The model under review builds one solid part; all positions refer to its coordinate system, in mm. A direction names the side the tool comes from. Round coordinates to 2 decimals unless told otherwise and drop trailing zeros. Write each loop counter-clockwise with the first axis right and the second up, starting at its lowest first coordinate (ties: lowest second). Pieces come first, ordered by that corner, then holes. Notation, with made-up numbers: M 74,13 L 95,13 A21 cw 95,28 Z; hole C 37,73 d3. An arc over 180 degrees is marked long. One line per item, written item: value. Start each with the question number.
1) For P1, Ø2, axis at y = -4, z = 2, coming from the -X side; P2, Ø1.5, axis at x = -11, z = 2, coming from the -Y side; P3, Ø1.5, axis at x = -20, z = 5, coming from the -Y side, all flat-tipped, find the tip position at first contact; note any pin that passes through.
2) Take a section at B-B, the plane y = -20.5. Write out the cut boundary in (x, z), and give its area (3 significant figures).
3) Take a section at D-D, the plane y = 13. Write out the cut boundary in (x, z), and give its area (3 significant figures).
4) Take a section at C-C, the plane z = 4. Write out the cut boundary in (x, y).
5) Wall thickness on probe 1 along X at (y, z) = (-19, 1.5); probe 2 along X at (y, z) = (-24.5, 5); probe 3 along Y at (x, z) = (0, 4.5): over which ranges is each line inside the solid? List them lowest first.
6) Mouldability with a two-part tool opening along Y and no side actions: class faces 1 (the face through (-3, -13, 7)), 2 (the face through (41.56, -23.91, 3.45)), 3 (the face through (-1.313, 29.172, 3.451)), 4 (the face through (15.219, -11.103, 3.451)) as +Y half, -Y half, draft (parallel to the pull), parting line (faces both ways), or undercut.
7) Take a section at A-A, the plane x = 16.5. Write out the cut boundary in (y, z), and give its area (3 significant figures).
8) Tool access review of faces 5 (the face through (13.575, 7.697, 3.451)), 6 (the face through (0.18, -10.75, 3.45)): name each direction out of +Z, -Z, +X, -X, +Y, -Y from which nothing blocks a thin tool from reaching the whole face with its end or side.
from build123d import *

# Parameters (mm, degrees)
F0_R        = 5.7
F1_DEPTH    = 7
F2_T1_DEPTH = 7


# Not quite as in the source:
# - a fillet or chamfer that OpenCascade refuses, or shapes differently, is made with other operations: its cross-section is extruded or revolved along the edge and cut away or added


with BuildPart() as f1:
    # F0 (on Top) → F1 (new body)
    with BuildSketch(Plane.XY):
        with BuildLine():
            ThreePointArc((35.7857254885, -10.7114257283), (13.3672908486, 8.0601420356), (8.7727432709, 36.9365701488))
            ThreePointArc((8.7727432709, 36.9365701488), (-0.3049324387, 47.9411231542), (-8.6164959528, 36.3470602301))
            ThreePointArc((-8.6164959528, 36.3470602301), (-13.6639331853, 7.5463424369), (-36.374379713, -10.8708665409))
            ThreePointArc((-36.374379713, -10.8708665409), (-41.3657643181, -24.2346408155), (-27.1692295357, -25.6356345017))
            ThreePointArc((-27.1692295357, -25.6356345017), (0.2966423367, -15.6064844725), (27.6016364421, -26.0657036079))
            ThreePointArc((27.6016364421, -26.0657036079), (41.6706967568, -23.7064823387), (35.7857254885, -10.7114257283))
        make_face()
        with Locations((-33.7284768728, -19.4731452019)):
            Circle(F0_R, mode=Mode.SUBTRACT)
        with Locations((33.7284768728, -19.4731452019)):
            Circle(F0_R, mode=Mode.SUBTRACT)
        with BuildLine():
            ThreePointArc((4.7464996897, 9.6453740568), (9.1265374503, 5.6805645994), (10.75, 0))
            ThreePointArc((10.75, 0), (10.7467864276, -0.2628335582), (10.7371476318, -0.5255099751))
            ThreePointArc((10.7371476318, -0.5255099751), (18.1244877352, -7.9521533479), (27.0404212358, -13.4506945549))
            ThreePointArc((27.0404212358, -13.4506945549), (26.0732155549, -14.7406010495), (25.3516724639, -16.1823781342))
            ThreePointArc((25.3516724639, -16.1823781342), (16.0918632419, -11.4192065952), (5.9798891173, -8.9332763388))
            ThreePointArc((5.9798891173, -8.9332763388), (0.0934488338, -10.749593821), (-5.8236788043, -9.0358876257))
            ThreePointArc((-5.8236788043, -9.0358876257), (-15.9490106817, -11.7201901353), (-25.168853801, -16.6923444418))
            ThreePointArc((-25.168853801, -16.6923444418), (-25.8023427534, -15.2097665041), (-26.6901867898, -13.864003315))
            ThreePointArc((-26.6901867898, -13.864003315), (-17.9352546235, -8.2263590641), (-10.726388807, -0.712097718))
            ThreePointArc((-10.726388807, -0.712097718), (-9.3561457462, 5.2938678465), (-4.9134688275, 9.5613976008))
            ThreePointArc((-4.9134688275, 9.5613976008), (-2.1754770535, 19.6723434832), (-1.8715674348, 30.1430389967))
            ThreePointArc((-1.8715674348, 30.1430389967), (-0.2708728015, 29.9503675537), (1.3385143259, 30.0463814492))
            ThreePointArc((1.3385143259, 30.0463814492), (1.8433913815, 19.6455656593), (4.7464996897, 9.6453740568))
        make_face(mode=Mode.SUBTRACT)
        with Locations((0, 38.9462904038)):
            Circle(F0_R, mode=Mode.SUBTRACT)
    extrude(amount=F1_DEPTH)

    # F2: fillet of radius 2 on 6 edges, made by hand

    # F2_s2 → F2_t1 (join)
    with BuildSketch(Plane.XY):
        with BuildLine():
            ThreePointArc((1.2437301381, 27.9302712072), (0.7204204263, 29.321617428), (-0.6184050998, 29.9675613661))
            ThreePointArc((-0.6184050998, 29.9675613661), (0.362205019, 29.9535818283), (1.3385143259, 30.0463814492))
            ThreePointArc((1.3385143259, 30.0463814492), (1.278556326, 28.9888891766), (1.2437301381, 27.9302712072))
        make_face()
        with BuildLine():
            ThreePointArc((0.2214111543, 29.9490143104), (-1.1869742591, 29.3190857733), (-1.7279638998, 27.8742018185))
            ThreePointArc((-1.7279638998, 27.8742018185), (-1.7853057388, 29.0095356327), (-1.8715674348, 30.1430389967))
            ThreePointArc((-1.8715674348, 30.1430389967), (-0.8307618987, 29.984714947), (0.2214111543, 29.9490143104))
        make_face()
        with BuildLine():
            ThreePointArc((23.566459331, -15.0422374987), (25.0330553595, -15.2847111045), (26.2618719824, -14.4482261568))
            ThreePointArc((26.2618719824, -14.4482261568), (25.7594602881, -15.290469662), (25.3516724639, -16.1823781342))
            ThreePointArc((25.3516724639, -16.1823781342), (24.4658362914, -15.6017068468), (23.566459331, -15.0422374987))
        make_face()
        with BuildLine():
            ThreePointArc((25.825901634, -15.1662548395), (25.9845602249, -13.6315930247), (25.0037488349, -12.4406402752))
            ThreePointArc((25.0037488349, -12.4406402752), (26.0156476793, -12.958647693), (27.0404212358, -13.4506945549))
            ThreePointArc((27.0404212358, -13.4506945549), (26.3829058187, -14.2728965647), (25.825901634, -15.1662548395))
        make_face()
        with BuildLine():
            ThreePointArc((-25.6434668826, -15.5193352093), (-25.7534757858, -14.0369063234), (-24.8101894691, -12.8880337086))
            ThreePointArc((-24.8101894691, -12.8880337086), (-25.7443926174, -13.3871823298), (-26.6901867898, -13.864003315))
            ThreePointArc((-26.6901867898, -13.864003315), (-26.1216653071, -14.6631121663), (-25.6434668826, -15.5193352093))
        make_face()
        with BuildLine():
            ThreePointArc((-26.0473127882, -14.7827594709), (-24.7975859659, -15.6874927486), (-23.2757849351, -15.4335615433))
            ThreePointArc((-23.2757849351, -15.4335615433), (-24.2303419405, -16.0508879397), (-25.168853801, -16.6923444418))
            ThreePointArc((-25.168853801, -16.6923444418), (-25.55214392, -15.7118183822), (-26.0473127882, -14.7827594709))
        make_face()
    extrude(amount=F2_T1_DEPTH)


solid = f1.part
Checked values:
1. P1: stops at x = -25.02
1. P2: stops at y = -17.28
1. P3: stops at y = -21.11
2. outline: M -42.67,0 L -39.34,0 L -39.34,7 L -42.67,7 Z; M -28.12,0 L -19.64,0 L -19.64,7 L -28.12,7 Z; M 19.58,0 L 28.12,0 L 28.12,7 L 19.58,7 Z; M 39.34,0 L 42.67,0 L 42.67,7 L 39.34,7 Z
2. area: 166 mm2
3. outline: M -10.97,0 L -3.69,0 L -3.69,7 L -10.97,7 Z; M 3.49,0 L 10.98,0 L 10.98,7 L 3.49,7 Z
3. area: 103 mm2
4. outline: M -36.37,-10.87 A9 ccw long -27.17,-25.64 A41.73 cw 27.6,-26.07 A9 ccw long 35.79,-10.71 A41.73 cw 8.77,36.94 A9 ccw long -8.62,36.35 A41.73 cw Z; hole C -33.73,-19.47 d11.4; hole M -25.79,-15.12 A2 ccw -23.28,-15.43 A44.6 cw -5.82,-9.04 A10.75 ccw 5.98,-8.93 A44.6 cw 23.57,-15.04 A2 ccw 25.99,-14.77 A2 ccw 25,-12.44 A44.6 cw 10.74,-0.53 A10.75 ccw 4.75,9.65 A44.6 cw 1.24,27.93 A2 ccw -0.2,29.89 A2 ccw -1.73,27.87 A44.6 cw -4.91,9.56 A10.75 ccw -10.73,-0.71 A44.6 cw -24.81,-12.89 A2 ccw Z; hole C 0,38.95 d11.4; hole C 33.73,-19.47 d11.4
5. probe 1: x = -42.72 to -39.41, -28.05 to -16.52, 16.46 to 28.05, 39.41 to 42.72
5. probe 2: x = -41.19 to -36.42, -31.04 to -25.78, 25.72 to 31.04, 36.42 to 41.19
5. probe 3: y = -15.61 to -10.75, 29.82 to 33.25, 44.65 to 47.95
6. face 1: draft
6. face 2: parting line
6. face 3: undercut
6. face 4: undercut
7. outline: M -19.02,0 L -11.57,0 L -11.57,7 L -19.02,7 Z; M -6.6,0 L 3.32,0 L 3.32,7 L -6.6,7 Z
7. area: 122 mm2
8. face 5: +Z, -Z, +X
8. face 6: +Z, -Z
